The model under review builds one solid part; all positions refer to its coordinate system, in mm. Coordinates: 2 decimals unless noted, no trailing zeros. Order: outer loops, then holes, each group sorted by start corner. A loop starts at its lowest first (then second) coordinate and runs counter-clockwise, first axis right, second up. Notation, with made-up numbers: M 12,60.5 L 58,60.5 A18 cw 58,83.5 Z; hole C 20,82.25 d4. An arc over 180 degrees is marked long. Answer in a Markdown table with one row per item.
from build123d import *

# Parameters (mm, degrees)
MASTER_SKETCH_W         = 635.3556
MASTER_SKETCH_H         = 498.348
BOSS_EXTRUDE1_DEPTH     = 3.175
SKETCH2_W               = 31.75
SKETCH2_H               = 190.5
BOSS_EXTRUDE2_DEPTH     = 3.175
M6_CLEARANCE_HOLE1_D    = 6.6
SKETCH5_W               = 2.286
SKETCH5_H               = 69.85
CUT_EXTRUDE1_DEPTH      = 430.182420788
LPATTERN1_COUNT         = 5
LPATTERN1_PITCH         = 98.8568
SKETCH7_W               = 254
SKETCH7_H               = 2.286
CUT_EXTRUDE3_DEPTH      = 430.182420788
LPATTERN2_COUNT         = 4
LPATTERN2_PITCH         = 98.8568
MIRROR4_COPY_1_SKETCH_W = 254
MIRROR4_COPY_1_SKETCH_H = 2.286
MIRROR4_COPY_1_DEPTH    = 430.182420788
MIRROR4_COPY_2_SKETCH_W = 254
MIRROR4_COPY_2_SKETCH_H = 2.286
MIRROR4_COPY_2_DEPTH    = 430.182420788
MIRROR4_COPY_3_SKETCH_W = 254
MIRROR4_COPY_3_SKETCH_H = 2.286
MIRROR4_COPY_3_DEPTH    = 430.182420788
SKETCH10_W              = 127
SKETCH10_H              = 31.75
BOSS_EXTRUDE3_DEPTH     = 3.175
M6_CLEARANCE_HOLE2_D    = 6.6
SKETCH6_W               = 254
SKETCH6_H               = 3.175
SKETCH6_W_2             = 147.1549
CUT_EXTRUDE2_DEPTH      = 449.361641774


with BuildPart() as part:
    # Master Sketch → Boss-Extrude1 (new body)
    with BuildSketch(Plane.XY):
        Rectangle(MASTER_SKETCH_W, MASTER_SKETCH_H)
    extrude(amount=BOSS_EXTRUDE1_DEPTH)

    # Sketch2 → Boss-Extrude2 (add)
    with BuildSketch(Plane.XY.offset(3.175)):
        with Locations((-333.5528, -153.924)):
            Rectangle(SKETCH2_W, SKETCH2_H)
    boss_extrude2 = extrude(amount=-BOSS_EXTRUDE2_DEPTH)

    # M6 Clearance Hole1 (through all)
    with Locations(Plane.XY.offset(3.175)):
        with Locations((-333.5528, -90.424), (-333.5528, -153.924), (-333.5528, -217.424)):
            m6_clearance_hole1 = Hole(M6_CLEARANCE_HOLE1_D / 2)

    # Mirror1: Boss-Extrude2, M6 Clearance Hole1 across plane
    add(boss_extrude2.mirror(Plane(origin=(0, 0, 0), x_dir=(0, 0, 1), z_dir=(1, 0, 0))))
    add(m6_clearance_hole1.mirror(Plane(origin=(0, 0, 0), x_dir=(0, 0, 1), z_dir=(1, 0, 0))), mode=Mode.SUBTRACT)

    # Sketch5 → Cut-Extrude1 (cut, through all)
    with BuildSketch(Plane.XY.offset(3.175)):
        with Locations((0, 197.7136)):
            Rectangle(SKETCH5_W, SKETCH5_H)
    cut_extrude1 = extrude(amount=-CUT_EXTRUDE1_DEPTH, mode=Mode.SUBTRACT)

    # LPattern1: Cut-Extrude1 ×5
    with Locations(*[(0, -i * LPATTERN1_PITCH, 0) for i in range(1, LPATTERN1_COUNT)]):
        add(cut_extrude1, mode=Mode.SUBTRACT)

    # Sketch7 → Cut-Extrude3 (cut, through all)
    with BuildSketch(Plane.XY.offset(3.175)):
        with Locations((-157.8229, 148.2852)):
            Rectangle(SKETCH7_W, SKETCH7_H)
    cut_extrude3 = extrude(amount=-CUT_EXTRUDE3_DEPTH, mode=Mode.SUBTRACT)

    # LPattern2: Cut-Extrude3 ×4
    with Locations(*[(0, -i * LPATTERN2_PITCH, 0) for i in range(1, LPATTERN2_COUNT)]):
        add(cut_extrude3, mode=Mode.SUBTRACT)

    # Mirror4: Cut-Extrude3 across plane
    add(cut_extrude3.mirror(Plane(origin=(0, 0, 0), x_dir=(0, 0, 1), z_dir=(1, 0, 0))), mode=Mode.SUBTRACT)

    # Mirror4 copy 1 sketch → Mirror4 copy 1 (cut, through all)
    with BuildSketch(Plane(origin=(0, -98.8568, 3.175), x_dir=(-1, 0, 0), z_dir=(0, 0, 1))):
        with Locations((-157.8229, -148.2852)):
            Rectangle(MIRROR4_COPY_1_SKETCH_W, MIRROR4_COPY_1_SKETCH_H)
    extrude(amount=-MIRROR4_COPY_1_DEPTH, mode=Mode.SUBTRACT)

    # Mirror4 copy 2 sketch → Mirror4 copy 2 (cut, through all)
    with BuildSketch(Plane(origin=(0, -197.7136, 3.175), x_dir=(-1, 0, 0), z_dir=(0, 0, 1))):
        with Locations((-157.8229, -148.2852)):
            Rectangle(MIRROR4_COPY_2_SKETCH_W, MIRROR4_COPY_2_SKETCH_H)
    extrude(amount=-MIRROR4_COPY_2_DEPTH, mode=Mode.SUBTRACT)

    # Mirror4 copy 3 sketch → Mirror4 copy 3 (cut, through all)
    with BuildSketch(Plane(origin=(0, -296.5704, 3.175), x_dir=(-1, 0, 0), z_dir=(0, 0, 1))):
        with Locations((-157.8229, -148.2852)):
            Rectangle(MIRROR4_COPY_3_SKETCH_W, MIRROR4_COPY_3_SKETCH_H)
    extrude(amount=-MIRROR4_COPY_3_DEPTH, mode=Mode.SUBTRACT)

    # Sketch10 → Boss-Extrude3 (add)
    with BuildSketch(Plane.XY.offset(3.175)):
        with Locations((-254.1778, 265.049)):
            Rectangle(SKETCH10_W, SKETCH10_H)
    boss_extrude3 = extrude(amount=-BOSS_EXTRUDE3_DEPTH)

    # M6 Clearance Hole2 (through all)
    with Locations(Plane.XY.offset(3.175)):
        with Locations((-285.9278, 265.049), (-222.4278, 265.049)):
            m6_clearance_hole2 = Hole(M6_CLEARANCE_HOLE2_D / 2)

    # Mirror6: Boss-Extrude3, M6 Clearance Hole2 across plane
    add(boss_extrude3.mirror(Plane(origin=(0, 0, 0), x_dir=(0, 0, 1), z_dir=(1, 0, 0))))
    add(m6_clearance_hole2.mirror(Plane(origin=(0, 0, 0), x_dir=(0, 0, 1), z_dir=(1, 0, 0))), mode=Mode.SUBTRACT)

    # Sketch6 → Cut-Extrude2 (cut, through all)
    with BuildSketch(Plane.XY.offset(3.175)):
        with Locations((-157.8229, -247.5865)):
            Rectangle(SKETCH6_W, SKETCH6_H)
        with Locations((157.8229, -247.5865)):
            Rectangle(SKETCH6_W, SKETCH6_H)
        with Locations((-104.40035, 247.5865)):
            Rectangle(SKETCH6_W_2, SKETCH6_H)
        with Locations((104.40035, 247.5865)):
            Rectangle(SKETCH6_W_2, SKETCH6_H)
    extrude(amount=-CUT_EXTRUDE2_DEPTH, mode=Mode.SUBTRACT)


solid = part.part
(1) To check wall thickness, follow line 1 (Y direction, x = 163.5, z = 0.9); line 2 (X direction, y = -216.5, z = 0.95); line 3 (Y direction, x = 197.5, z = 2.9). State the ranges of each line that lie inside material, in increasing order. Write a range as [from, to].
Report:
| item | result |
|---|---|
| line 1 | [-246, -149.43], [-147.14, -50.57], [-48.29, 48.29], [50.57, 147.14], [149.43, 246] |
| line 2 | [-349.43, -336.72], [-330.38, -1.14], [1.14, 330.38], [336.72, 349.43] |
| line 3 | [-246, -149.43], [-147.14, -50.57], [-48.29, 48.29], [50.57, 147.14], [149.43, 280.92] |
(2) Take a section at B-B (y = 179.5). Write out the cut boundary in (x, z) (3 decimals).
Report:
| item | result |
|---|---|
| outline | M -317.678,0 L -1.143,0 L -1.143,3.175 L -317.678,3.175 Z; M 1.143,0 L 317.678,0 L 317.678,3.175 L 1.143,3.175 Z |
(3) Take a section at D-D (x = 18). Write out the cut boundary in (y, z) (3 decimals).
Report:
| item | result |
|---|---|
| outline | M -249.174,0 L 249.174,0 L 249.174,3.175 L -249.174,3.175 Z |
(4) Take a section at A-A (x = -80.5). Write out the cut boundary in (y, z) (3 decimals).
Report:
| item | result |
|---|---|
| outline | M -245.999,0 L -149.428,0 L -149.428,3.175 L -245.999,3.175 Z; M -147.142,0 L -50.571,0 L -50.571,3.175 L -147.142,3.175 Z; M -48.285,0 L 48.285,0 L 48.285,3.175 L -48.285,3.175 Z; M 50.571,0 L 147.142,0 L 147.142,3.175 L 50.571,3.175 Z; M 149.428,0 L 245.999,0 L 245.999,3.175 L 149.428,3.175 Z |
(5) Take a section at C-C (z = 1.55). State how many separate pieces and enclosed holes the cut face has, then the cut area to 3 significant figures.
Report:
| item | result |
|---|---|
| separate pieces | 1 |
| enclosed holes | 23 |
| area | 328,000 mm^2 |
(6) Insertion check: P1, Ø1, axis at x = 326, z = 1, coming from the +Y side; P2, Ø1.6, axis at y = 108, z = 2, coming from the -X side; P3, Ø1, axis at x = -183.5, z = 1.5, coming from the +Y side. Each pin has a flat end and moves straight along its axis. Give the tip position at first contact, or say it passes through.
Report:
| item | result |
|---|---|
| P1 | y = -58.67 |
| P2 | x = -317.68 |
| P3 | y = 249.17 |
